from build123d import *

# Parameters (mm, degrees)
NUT_CLIP_BLANK_SKETCH_W     = 6.6
NUT_CLIP_BLANK_SKETCH_H     = 13
NUT_CLIP_BLANK_DEPTH        = 14
M6_NUT_CLEARANCE_DEPTH      = 5.3
LOAD_WASHER_RELIEF_SKETCH_R = 6.2
LOAD_WASHER_RELIEF_DEPTH    = 1.9


with BuildPart() as part:
    # Nut clip blank sketch → Nut clip blank (new body)
    with BuildSketch(Plane.XY.offset(-27)):
        with Locations((44.408348754, -29)):
            Rectangle(NUT_CLIP_BLANK_SKETCH_W, NUT_CLIP_BLANK_SKETCH_H)
    extrude(amount=NUT_CLIP_BLANK_DEPTH)

    # M6 nut clearance sketch → M6 nut clearance (cut)
    with BuildSketch(Plane(origin=(41.008348754, 0, 0), x_dir=(0, 0, -1), z_dir=(1, 0, 0))):
        Polygon((16.4977786, -23.8), (13.4955572, -29), (16.4977786, -34.2), (22.5022214, -34.2), (25.5044428, -29), (22.5022214, -23.8), align=None)
    extrude(amount=M6_NUT_CLEARANCE_DEPTH, mode=Mode.SUBTRACT)

    # Load washer relief sketch → Load washer relief (cut)
    with BuildSketch(Plane(origin=(46.008348754, 0, 0), x_dir=(0, 0, -1), z_dir=(1, 0, 0))):
        with Locations(Location((19.5, -29, 0), (0, 0, 180))):
            Circle(LOAD_WASHER_RELIEF_SKETCH_R)
    extrude(amount=LOAD_WASHER_RELIEF_DEPTH, mode=Mode.SUBTRACT)


solid = part.part
Design review of the part built by this model. Coordinates are the model's own, in mm. A direction names the side the tool comes from. Round coordinates to 2 decimals unless told otherwise and drop trailing zeros. Order: outer loops, then holes, each group sorted by start corner. A loop starts at its lowest first (then second) coordinate and runs counter-clockwise, first axis right, second up. Notation, with made-up numbers: M 26.5,-39.75 L 30.5,-39.75 A18 cw 30.5,-7.75 Z; hole C 11.5,14.25 d9. An arc over 180 degrees is marked long. Answer as CSV lines item,"result". Start each with the question number.
1) Add section B-B (x = 44.75). Give the boundary of the cut face in (y, z), then the cut area to 3 significant figures.
2) Add section C-C (y = -25.75). Give the boundary of the cut face in (x, z).
3) Tool access review of faces 5 (the face through (44, -34.2, -19)), 6 (the face through (46.008, -26, -24)), 7 (the face through (44, -29, -27)): name each direction out of +Z, -Z, +X, -X, +Y, -Y from which nothing blocks a thin tool from reaching the whole face with its end or side.
4) For pin 1 Ø6 at (y, z) = (-31, -18) entering from +X, flat-tipped, find the tip position at first contact; note if it passes through.
5) The part is to be moulded in two halves that separate along Z. For faces 1 (the face through (43.524, -26.436, -24.024)), 2 (the face through (44, -29, -13)), 3 (the face through (44, -22.5, -20)), 4 (the face through (44, -23.8, -20)), say which applies: +Z half, -Z half, draft (parallel to the pull), parting line (faces both ways), or undercut.
6) Wall thickness on line 1 along Y through (x, z) = (47.1, -19.5); line 2 along Z through (x, y) = (46.75, -29); line 3 along Y through (x, z) = (42.25, -19.75): over which ranges is each line inside the solid? List them lowest first. Write a range as [from, to].
7) Add section A-A (z = -24). Give the boundary of the cut face in (x, y), then the cut area to 3 significant figures.
Resolved:
1,outline,"M -35.5,-27 L -22.5,-27 L -22.5,-13 L -35.5,-13 Z; hole M -34.2,-22.5 L -29,-25.5 L -23.8,-22.5 L -23.8,-16.5 L -29,-13.5 L -34.2,-16.5 Z"
1,area,"88.3 mm^2"
2,outline,"M 41.11,-27 L 47.71,-27 L 47.71,-24.78 L 46.01,-24.78 L 46.01,-23.63 L 41.11,-23.63 Z; M 41.11,-15.37 L 46.01,-15.37 L 46.01,-14.22 L 47.71,-14.22 L 47.71,-13 L 41.11,-13 Z"
3,face 5,"+X, -X"
3,face 6,"+X"
3,face 7,"-Z, +X, -X, +Y, -Y"
4,pin 1,"x = 46.01"
5,face 1,"undercut"
5,face 2,"+Z half"
5,face 3,"draft"
5,face 4,"undercut"
6,line 1,"[-35.5, -35.2], [-22.8, -22.5]"
6,line 2,"[-27, -25.7], [-13.3, -13]"
6,line 3,"[-35.5, -34.2], [-23.8, -22.5]"
7,outline,"M 41.11,-35.5 L 47.71,-35.5 L 47.71,-33.26 L 46.01,-33.26 L 46.01,-31.61 L 41.11,-31.61 Z; M 41.11,-26.39 L 46.01,-26.39 L 46.01,-24.74 L 47.71,-24.74 L 47.71,-22.5 L 41.11,-22.5 Z"
7,area,"45.8 mm^2"
